Autodesk Fusion 360 part; units mm, degrees
sketch "Sketch1" plane through (0, 0, 0) normal (0, 0, 1) x (1, 0, 0)
  circle A0 centre (0, 0) radius 27.5
  circle A1 centre (30, -51.9615) radius 10
  line L0 (0, 0) -> (0, -67.6601)
  line L1 (0, 0) -> (30, -51.9615) construction
  line L2 (0, 0) -> (10.1597, -17.5971) construction
  line L3 (0, 0) -> (20.3193, 0) construction
  arc A2 (39.4278, -21.6899) -> (42.203, -38.7295) centre (51.6942, -28.4379) ccw
  arc A3 (14.5714, -61.2329) -> (42.203, -38.7295) centre (30, -51.9615) ccw
  circle A4 centre (-30, -51.9615) radius 10
  arc A5 (-42.203, -38.7295) -> (-39.4278, -21.6899) centre (-51.6942, -28.4379) ccw
  arc A6 (14.5714, -61.2329) -> (-14.5714, -61.2329) centre (0, -69.9893) ccw
  arc A7 (-42.203, -38.7295) -> (-14.5714, -61.2329) centre (-30, -51.9615) ccw
  arc A8 (-14.5714, 61.2329) -> (-42.203, 38.7295) centre (-30, 51.9615) ccw
  arc A9 (-39.4278, 21.6899) -> (-42.203, 38.7295) centre (-51.6942, 28.4379) ccw
  circle A10 centre (-30, 51.9615) radius 10
  arc A11 (-14.5714, 61.2329) -> (14.5714, 61.2329) centre (0, 69.9893) ccw
  arc A12 (42.203, 38.7295) -> (14.5714, 61.2329) centre (30, 51.9615) ccw
  circle A13 centre (30, 51.9615) radius 10
  arc A14 (42.203, 38.7295) -> (39.4278, 21.6899) centre (51.6942, 28.4379) ccw
  arc A15 (39.4278, -21.6899) -> (39.4278, 21.6899) centre (0, 0) ccw
  arc A16 (-39.4278, 21.6899) -> (-39.4278, -21.6899) centre (0, 0) ccw
  dimension "d1" = 55
  dimension "d2" = 90
  dimension "d4" = 20
  dimension "d5" = 36
  dimension "d6" = 28
  dimension "d7" = 60
  dimension "d8" = 34
extrude "Extrude1" add sketch "Sketch1" along normal blind 20
sketch "Sketch2" plane through (0, 0, 20) normal (0, 0, 1) x (-1, 0, 0)
  circle A0 centre (30, 51.9615) radius 10
  circle A1 centre (30, -51.9615) radius 10
  circle A2 centre (-30, -51.9615) radius 10
  circle A3 centre (-30, 51.9615) radius 10
  circle A4 centre (0, 0) radius 27.5
  arc A5 (14.5714, -61.2329) -> (42.203, -38.7295) centre (30, -51.9615) ccw
  arc A6 (39.4278, -21.6899) -> (42.203, -38.7295) centre (51.6942, -28.4379) ccw
  arc A7 (39.4278, -21.6899) -> (39.4278, 21.6899) centre (0, 0) ccw
  arc A8 (42.203, 38.7295) -> (39.4278, 21.6899) centre (51.6942, 28.4379) ccw
  arc A9 (42.203, 38.7295) -> (14.5714, 61.2329) centre (30, 51.9615) ccw
  arc A10 (-14.5714, 61.2329) -> (14.5714, 61.2329) centre (0, 69.9893) ccw
  arc A11 (-14.5714, 61.2329) -> (-42.203, 38.7295) centre (-30, 51.9615) ccw
  arc A12 (-39.4278, 21.6899) -> (-42.203, 38.7295) centre (-51.6942, 28.4379) ccw
  arc A13 (-39.4278, 21.6899) -> (-39.4278, -21.6899) centre (0, 0) ccw
  arc A14 (-42.203, -38.7295) -> (-39.4278, -21.6899) centre (-51.6942, -28.4379) ccw
  arc A15 (-42.203, -38.7295) -> (-14.5714, -61.2329) centre (-30, -51.9615) ccw
  arc A16 (14.5714, -61.2329) -> (-14.5714, -61.2329) centre (0, -69.9893) ccw
  circle A17 centre (0, 0) radius 27.5
  circle A18 centre (0, 0) radius 45
extrude "Extrude2" add sketch "Sketch2" along normal blind 3 contours A7 A13 A18
sketch "Sketch3" plane through (0, 0, 23) normal (0, 0, 1) x (-1, 0, 0)
  circle A0 centre (0, 0) radius 27.5
  circle A1 centre (0, 0) radius 45
  line L0 (0, 0) -> (45, 0) construction
  line L1 (45, 0) -> (45, -1)
  line L2 (44.7214, -5) -> (27.0416, -5)
  line L3 (44.7214, 5) -> (27.0416, 5)
  line L4 (26.6908, 36.2298) -> (17.8509, 20.9187)
  line L5 (18.0306, 41.2298) -> (9.1907, 25.9187)
  line L6 (-18.0306, 41.2298) -> (-9.1907, 25.9187)
  line L7 (-26.6908, 36.2298) -> (-17.8509, 20.9187)
  line L8 (-44.7214, 5) -> (-27.0416, 5)
  line L9 (-44.7214, -5) -> (-27.0416, -5)
  line L10 (-26.6908, -36.2298) -> (-17.8509, -20.9187)
  line L11 (-18.0306, -41.2298) -> (-9.1907, -25.9187)
  line L12 (18.0306, -41.2298) -> (9.1907, -25.9187)
  line L13 (26.6908, -36.2298) -> (17.8509, -20.9187)
  arc A2 (-9.1907, -25.9187) -> (9.1907, -25.9187) centre (0, 0) ccw
  arc A3 (-18.0306, -41.2298) -> (18.0306, -41.2298) centre (0, 0) ccw
  arc A4 (-44.7214, -5) -> (-26.6908, -36.2298) centre (0, 0) ccw
  arc A5 (-27.0416, -5) -> (-17.8509, -20.9187) centre (0, 0) ccw
  arc A6 (17.8509, -20.9187) -> (27.0416, -5) centre (0, 0) ccw
  arc A7 (26.6908, -36.2298) -> (44.7214, -5) centre (0, 0) ccw
  arc A8 (27.0416, 5) -> (17.8509, 20.9187) centre (0, 0) ccw
  arc A9 (9.1907, 25.9187) -> (-9.1907, 25.9187) centre (0, 0) ccw
  arc A10 (-17.8509, 20.9187) -> (-27.0416, 5) centre (0, 0) ccw
  arc A11 (-26.6908, 36.2298) -> (-44.7214, 5) centre (0, 0) ccw
  arc A12 (44.7214, 5) -> (26.6908, 36.2298) centre (0, 0) ccw
  arc A13 (18.0306, 41.2298) -> (-18.0306, 41.2298) centre (0, 0) ccw
  dimension "d15" = 360
extrude "Extrude3" add sketch "Sketch3" along normal blind 3 contours A0 A1 L3 L4 A8 A12 | A0 A1 L2 L13 A6 A7 | A0 A1 L5 L6 A9 A13 | A0 A1 L11 L12 A2 A3 | A0 A1 L7 L8 A10 A11 | A0 A1 L9 L10 A4 A5
Geometry check sheet. Reference: the model listing, model coordinates, mm. A direction names the side the tool comes from. Give positions to 0.01 mm unless a question says otherwise; leave off trailing zeros. Loops run counter-clockwise (first coordinate to the right, second up) from the corner with the lowest first, then second, coordinate; pieces in that order, holes last. Notation, with made-up numbers: M 22,28 L 47,28 A16 cw 47,40 Z; hole C 11.5,49.25 d10. An arc over 180 degrees is marked long. Write each question's results on one line, items separated by ' | '.
1) Section check C-C, the plane z = 14.5. Record the boundary of the cut face in (x, y), plus the area to 3 significant figures.
Answers follow:
outline: M -42.2,-38.73 A18 ccw long -14.57,-61.23 A17 cw 14.57,-61.23 A18 ccw long 42.2,-38.73 A14 cw 39.43,-21.69 A45 ccw 39.43,21.69 A14 cw 42.2,38.73 A18 ccw long 14.57,61.23 A17 cw -14.57,61.23 A18 ccw long -42.2,38.73 A14 cw -39.43,21.69 A45 ccw -39.43,-21.69 A14 cw Z; hole C -30,-51.96 d20; hole C -30,51.96 d20; hole C 0,0 d55; hole C 30,-51.96 d20; hole C 30,51.96 d20 | area: 7,370 mm2
2) Section check D-D, the plane x = 30. Record the boundary of the cut face in (y, z), plus the area to 3 significant figures.
Answers follow:
outline: M -69.96,0 L -61.96,0 L -61.96,20 L -69.96,20 Z; M -41.96,0 L 41.96,0 L 41.96,20 L 33.54,20 L 33.54,26 L 5,26 L 5,23 L -5,23 L -5,26 L -33.54,26 L -33.54,20 L -41.96,20 Z; M 61.96,0 L 69.96,0 L 69.96,20 L 61.96,20 Z | area: 2,370 mm2
3) Thickness scan on line 1 (Y direction, x = 30, z = 9); line 2 (Y direction, x = 0, z = 6.75); line 3 (X direction, y = 0, z = 10.75). Record the ranges inside material, lowest first.
Answers follow:
line 1: -69.96 to -61.96, -41.96 to 41.96, 61.96 to 69.96 | line 2: -52.99 to -27.5, 27.5 to 52.99 | line 3: -45 to -27.5, 27.5 to 45
4) Section check A-A, the plane x = -33. Record the boundary of the cut face in (y, z), plus the area to 3 significant figures.
Answers follow:
outline: M -69.71,0 L -61.5,0 L -61.5,20 L -69.71,20 Z; M -42.42,0 L 42.42,0 L 42.42,20 L 30.59,20 L 30.59,26 L 5,26 L 5,23 L -5,23 L -5,26 L -30.59,26 L -30.59,20 L -42.42,20 Z; M 61.5,0 L 69.71,0 L 69.71,20 L 61.5,20 Z | area: 2,360 mm2
5) Tool access check on faces 1 (the face through (-18, 31, 23)), 2 (the face through (-41.029, -66.187, 9.86)), 3 (the face through (-36, 5, 24)), 4 (the face through (0.25, 52.99, 9.86)), 5 (the face through (0.92, -44.99, 22.96)). Record the directions out of +Z, -Z, +X, -X, +Y, -Y that give a thin tool (end or side, any length) a straight path to the whole face; none if there is none.
Answers follow:
face 1: +Z | face 2: +Z, -Z | face 3: +Z, +X, -X | face 4: +Z, -Z, +Y | face 5: +Z, -Y
6) Gauge pin test, flat ends, axial feed: pin 1 (4 mm diameter, centred on y = -30, z = 21.5, fed in from -X); pin 2 (0.9 mm diameter, centred on x = 34.5, z = 24, fed in from -Y); pin 3 (1 mm diameter, centred on x = 37.5, z = 21, fed in from +Y); pin 4 (16 mm diameter, centred on x = -30, y = 51.96, fed in from +Z). Record the tip position at first contact, or that the pin passes through.
Answers follow:
pin 1: x = -37.99 | pin 2: y = -29.42 | pin 3: y = 25.61 | pin 4: through
7) Section check B-B, the plane y = -58.5. Record the boundary of the cut face in (x, z).
Answers follow:
outline: M -46.77,0 L -37.57,0 L -37.57,20 L -46.77,20 Z; M -22.43,0 L -12.53,0 L -12.53,20 L -22.43,20 Z; M 12.53,0 L 22.43,0 L 22.43,20 L 12.53,20 Z; M 37.57,0 L 46.77,0 L 46.77,20 L 37.57,20 Z
